Check sheet for the modelled part. Datum: model origin and axes. Units: mm. Face numbers are marked on the shaded views. A direction names the side the tool comes from. Give positions to 0.01 mm unless a question says otherwise; leave off trailing zeros. Write each loop counter-clockwise with the first axis right and the second up, starting at its lowest first coordinate (ties: lowest second). Pieces come first, ordered by that corner, then holes. Notation, with made-up numbers: M -36,17.5 L 0,17.5 A12 ccw 0,39.5 Z; hole C 83.25,12.25 d7. An arc over 180 degrees is marked long. Write item = value, one per line. Start each with the question number.
1) Cross-section at C-C, the plane x = -0.5. Record the cut outline in (y, z), plus the area to 3 significant figures.
2) Cross-section at A-A, the plane z = 6. Record the cut outline in (x, y).
3) Access from +Z, -Z, +X, -X, +Y, -Y to the whole of each face (thin tool, end or side, straight path). Record for the marked faces 1 and 2.
4) Cross-section at D-D, the plane y = 7.25. Record the cut outline in (x, z), plus the area to 3 significant figures.
5) Cross-section at B-B, the plane y = -6. Record the cut outline in (x, z).
6) Go/stop test with flat-tipped pins: pin 1 (1.5 mm diameter, centred on x = -12, y = -5, fed in from +Z); pin 2 (1.8 mm diameter, centred on y = -3.5, z = 6, fed in from +X); pin 3 (2 mm diameter, centred on y = -2.5, z = 2.5, fed in from +X). Record where each tip stops, or that it passes through.
7) Scan lines: line 1 along Y through (x, z) = (-16.65, 6); line 2 along Z through (x, y) = (-10, 7); line 3 along X through (y, z) = (5, 6.75). Record each from-to range of solid material in increasing order. Write a range as [from, to].
```python
from build123d import *

# Parameters (mm, degrees)
F_10_MM_EXTRUDE_DEPTH  = 10
F_8_START              = -8
SKETCH2_R              = 9.5
F_8_MM_CUT_DEPTH       = 8
SKETCH4_R              = 1.8
CUT_EXTRUDE_3_6D_DEPTH = 8
R2_FILET_R             = 2


with BuildPart() as part:
    # Sketch1 → 10 mm extrude (new body)
    with BuildSketch(Plane(origin=(0, 0, 0), x_dir=(0, 1, 0), z_dir=(0, 0, 1))):
        with BuildLine():
            Line((-11, 18), (-11, 0))
            ThreePointArc((-11, 0), (-7.778174593, 7.778174593), (0, 11))
            Line((0, 11), (0, 18))
            Line((0, 18), (-11, 18))
        make_face()
        with BuildLine():
            Line((0, 18), (0, 11))
            ThreePointArc((0, 11), (7.778174593, 7.778174593), (11, 0))
            Line((11, 0), (11, 18))
            Line((11, 18), (0, 18))
        make_face()
        with BuildLine():
            ThreePointArc((0, 11), (-7.778174593, 7.778174593), (-11, 0))
            Line((-11, 0), (-9.5, 0))
            ThreePointArc((-9.5, 0), (-6.717514421, 6.717514421), (0, 9.5))
            Line((0, 9.5), (0, 11))
        make_face()
        with BuildLine():
            Line((-9.5, 0), (-11, 0))
            ThreePointArc((-11, 0), (-7.778174593, -7.778174593), (0, -11))
            Line((0, -11), (0, -9.5))
            ThreePointArc((0, -9.5), (-6.717514421, -6.717514421), (-9.5, 0))
        make_face()
        with BuildLine():
            ThreePointArc((11, 0), (7.778174593, 7.778174593), (0, 11))
            Line((0, 11), (0, 9.5))
            ThreePointArc((0, 9.5), (6.717514421, 6.717514421), (9.5, 0))
            Line((9.5, 0), (11, 0))
        make_face()
        with BuildLine():
            Line((0, -9.5), (0, -11))
            ThreePointArc((0, -11), (7.778174593, -7.778174593), (11, 0))
            Line((11, 0), (9.5, 0))
            ThreePointArc((9.5, 0), (6.717514421, -6.717514421), (0, -9.5))
        make_face()
    extrude(amount=F_10_MM_EXTRUDE_DEPTH)

    # Sketch2 → 8 mm cut (cut)
    with BuildSketch(Plane(origin=(0, 0, 10), x_dir=(0, -1, 0), z_dir=(0, 0, 1)).offset(F_8_START)):
        with BuildLine():
            Line((11, -15), (11, 0))
            ThreePointArc((11, 0), (0, 11), (-11, 0))
            Line((-11, 0), (-11, -15))
            Line((-11, -15), (11, -15))
        make_face()
        with Locations(Location((0, 0, 0), (0, 0, 90))):
            Circle(SKETCH2_R, mode=Mode.SUBTRACT)
    extrude(amount=F_8_MM_CUT_DEPTH, mode=Mode.SUBTRACT)

    # Sketch4 → Cut-Extrude 3.6D (cut)
    with BuildSketch(Plane.YZ.offset(-15)):
        with Locations(Location((-0.001698954, 6, 0), (0, 0, 270))):
            Circle(SKETCH4_R)
    extrude(amount=-CUT_EXTRUDE_3_6D_DEPTH, mode=Mode.SUBTRACT)

    # R2 Filet
    r2_filet_edges = [part.edges().sort_by_distance(p)[0] for p in [
        (-15, 0, 2),
        (-18, 0, 0),
    ]]
    fillet(r2_filet_edges, radius=R2_FILET_R)


solid = part.part
```
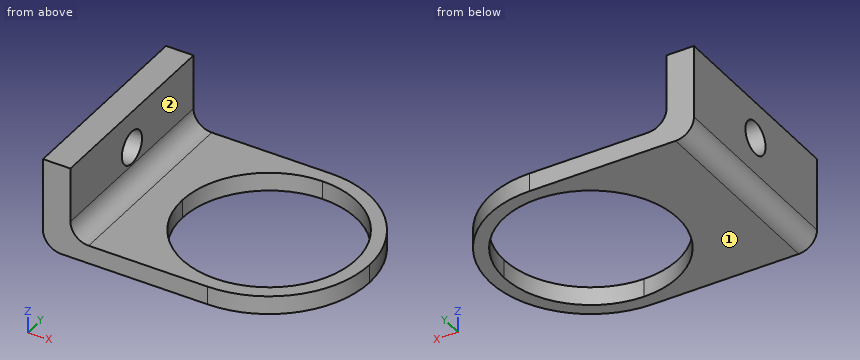
Reply:
q1.outline = M -11,0 L -9.49,0 L -9.49,2 L -11,2 Z; M 9.49,0 L 11,0 L 11,2 L 9.49,2 Z
q1.area = 6.05 mm2
q2.outline = M -18,-11 L -15,-11 L -15,-1.8 L -18,-1.8 Z; M -18,1.8 L -15,1.8 L -15,11 L -18,11 Z
q3.face_1 = -Z, +X, -X, +Y, -Y
q3.face_2 = +Z, +X, +Y, -Y
q4.outline = M -18,2 A2 ccw -16,0 L -6.14,0 L -6.14,2 L -13,2 A2 cw -15,4 L -15,10 L -18,10 Z; M 6.14,0 L 8.27,0 L 8.27,2 L 6.14,2 Z
q4.area = 52.0 mm2
q5.outline = M -18,2 A2 ccw -16,0 L -7.37,0 L -7.37,2 L -13,2 A2 cw -15,4 L -15,10 L -18,10 Z; M 7.37,0 L 9.22,0 L 9.22,2 L 7.37,2 Z
q6.pin_1 = 2
q6.pin_2 = -15
q6.pin_3 = 10.88
q7.line_1 = [-11, -1.8], [1.8, 11]
q7.line_2 = [0, 2]
q7.line_3 = [-18, -15]
